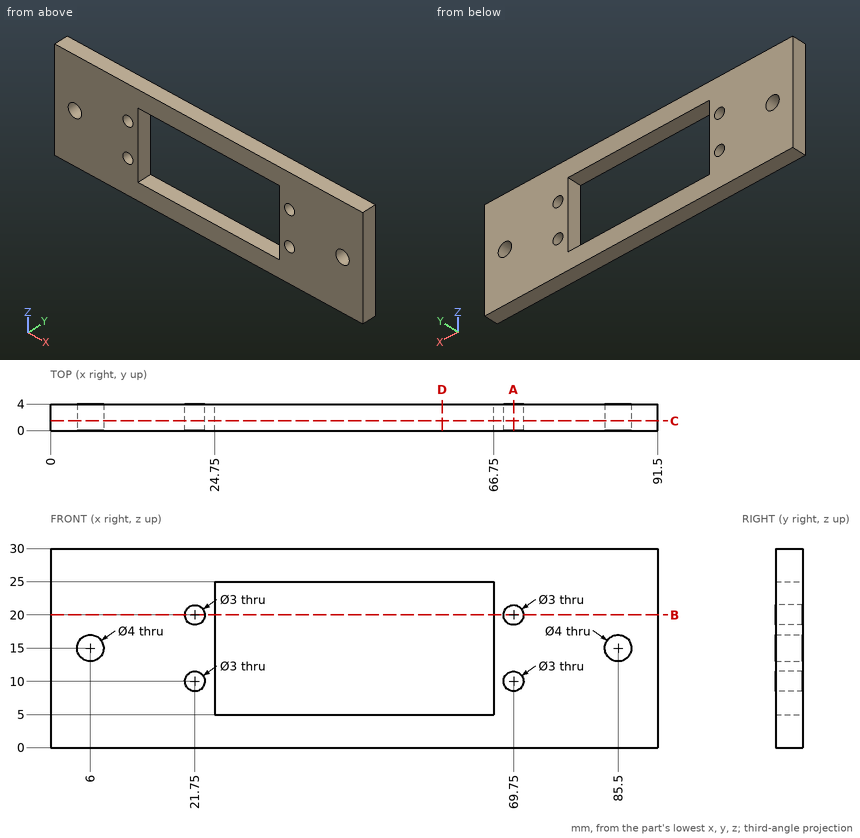
Source: three-view drawing plus pictorial views. Frame: mm from the lowest corner of the part. Give positions to 0.01 mm unless a question says otherwise; leave off trailing zeros. Order: outer loops, then holes, each group sorted by start corner. A loop starts at its lowest first (then second) coordinate and runs counter-clockwise, first axis right, second up. Notation, with made-up numbers: (56, 32) -> (74, 32) arc R22 cw to (74, 40) -> close; hole circle Ø2 at (36.5, 62). An arc over 180 degrees is marked (long way). Put each result on its own line as item: value.
Q1. Section C-C, the plane y = 1.45. Return loops of the section in (x, z), then the cut area to 3 significant figures.
Here are the results:
outline: (0, 0) -> (91.5, 0) -> (91.5, 30) -> (0, 30) -> close; hole circle Ø4 at (6, 15); hole circle Ø3 at (21.75, 10); hole circle Ø3 at (21.75, 20); hole (24.75, 5) -> (66.75, 5) -> (66.75, 25) -> (24.75, 25) -> close; hole circle Ø3 at (69.75, 10); hole circle Ø3 at (69.75, 20); hole circle Ø4 at (85.5, 15)
area: 1,850 mm^2
Q2. Material intervals for L1, parallel to X at y = 1.55, z = 15; L2, parallel to X at y = 2.5, z = 10; L3, parallel to Z at x = 69.75, y = 2.6, sorted ascending.
Here are the results:
L1: x = 0 to 4, 8 to 24.75, 66.75 to 83.5, 87.5 to 91.5
L2: x = 0 to 20.25, 23.25 to 24.75, 66.75 to 68.25, 71.25 to 91.5
L3: z = 0 to 8.5, 11.5 to 18.5, 21.5 to 30
Q3. Section B-B, the plane z = 20. Return loops of the section in (x, y), then the cut area to 3 significant figures.
Here are the results:
outline: (0, 0) -> (20.25, 0) -> (20.25, 4) -> (0, 4) -> close; (23.25, 0) -> (24.75, 0) -> (24.75, 4) -> (23.25, 4) -> close; (66.75, 0) -> (68.25, 0) -> (68.25, 4) -> (66.75, 4) -> close; (71.25, 0) -> (91.5, 0) -> (91.5, 4) -> (71.25, 4) -> close
area: 174 mm^2
Q4. Section A-A, the plane x = 69.75. Return loops of the section in (y, z).
Here are the results:
outline: (0, 0) -> (4, 0) -> (4, 8.5) -> (0, 8.5) -> close; (0, 11.5) -> (4, 11.5) -> (4, 18.5) -> (0, 18.5) -> close; (0, 21.5) -> (4, 21.5) -> (4, 30) -> (0, 30) -> close
Q5. Section D-D, the plane x = 59. Return loops of the section in (y, z).
Here are the results:
outline: (0, 0) -> (4, 0) -> (4, 5) -> (0, 5) -> close; (0, 25) -> (4, 25) -> (4, 30) -> (0, 30) -> close
